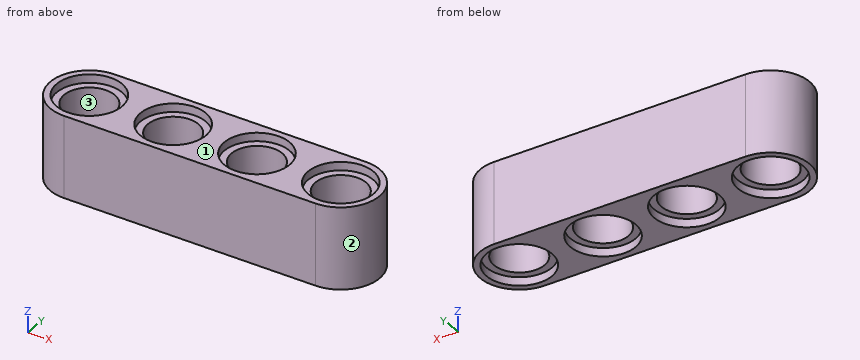
from build123d import *

# Parameters (mm, degrees)
BOSS_EXTRUDE1_DEPTH = 7.76
SKETCH2_R           = 3.1
CUT_EXTRUDE1_DEPTH  = 0.8
SKETCH3_R           = 2.4
CUT_EXTRUDE2_DEPTH  = 93.711483407
CUT_EXTRUDE3_START  = -0.8
SKETCH4_R           = 3.1
CUT_EXTRUDE3_DEPTH  = 0.8


with BuildPart() as part:
    # Sketch1 → Boss-Extrude1 (new body)
    with BuildSketch(Plane.XY):
        with BuildLine():
            Line((-88.686195286, 3.69), (-64.766195286, 3.69))
            ThreePointArc((-64.766195286, 3.69), (-61.076195286, 0), (-64.766195286, -3.69))
            Line((-64.766195286, -3.69), (-88.686195286, -3.69))
            ThreePointArc((-88.686195286, -3.69), (-92.376195286, 0), (-88.686195286, 3.69))
        make_face()
    extrude(amount=BOSS_EXTRUDE1_DEPTH)

    # Sketch2 → Cut-Extrude1 (cut)
    with BuildSketch(Plane(origin=(0, 0, 0), x_dir=(-1, 0, 0), z_dir=(0, 0, -1))):
        with Locations((64.766195286, 0)):
            Circle(SKETCH2_R)
        with Locations((72.736195286, 0)):
            Circle(SKETCH2_R)
        with Locations((80.706195286, 0)):
            Circle(SKETCH2_R)
        with Locations((88.676195286, 0)):
            Circle(SKETCH2_R)
    extrude(amount=-CUT_EXTRUDE1_DEPTH, mode=Mode.SUBTRACT)

    # Sketch3 → Cut-Extrude2 (cut, through all)
    with BuildSketch(Plane(origin=(0, 0, 0.8), x_dir=(-1, 0, 0), z_dir=(0, 0, -1))):
        with Locations((64.766195286, 0)):
            Circle(SKETCH3_R)
        with Locations((72.736195286, 0)):
            Circle(SKETCH3_R)
        with Locations((80.706195286, 0)):
            Circle(SKETCH3_R)
        with Locations((88.676195286, 0)):
            Circle(SKETCH3_R)
    extrude(amount=-CUT_EXTRUDE2_DEPTH, mode=Mode.SUBTRACT)

    # Sketch4 → Cut-Extrude3 (cut)
    with BuildSketch(Plane.XY.offset(7.76).offset(CUT_EXTRUDE3_START)):
        with Locations(Location((-88.676195286, 0, 0), (0, 0, 180))):
            Circle(SKETCH4_R)
        with Locations(Location((-80.706195286, 0, 0), (0, 0, 180))):
            Circle(SKETCH4_R)
        with Locations(Location((-72.736195286, 0, 0), (0, 0, 180))):
            Circle(SKETCH4_R)
        with Locations(Location((-64.766195286, 0, 0), (0, 0, 180))):
            Circle(SKETCH4_R)
    extrude(amount=CUT_EXTRUDE3_DEPTH, mode=Mode.SUBTRACT)


solid = part.part
Part model, mm, in its own coordinate system. Face numbers are marked on the shaded views. Round coordinates to 2 decimals unless told otherwise and drop trailing zeros. Write each loop counter-clockwise with the first axis right and the second up, starting at its lowest first coordinate (ties: lowest second). Pieces come first, ordered by that corner, then holes. Notation, with made-up numbers: M 14,42.5 L 73,42.5 A31 ccw 73,66.5 Z; hole C 25.25,56 d8. An arc over 180 degrees is marked long. Return JSON: item names as keys, results as strings. Group by question number.
(1) Saw through at A-A on z = 3.5. Write the cut outline in (x, y), then the cut area to 3 significant figures.
(2) Drill centre lines: probe 1 along X at (y, z) = (-1, 6.25); probe 2 along Z at (x, y) = (-73, -3); probe 3 along X at (y, z) = (2, 1.5). Where is each one in solid material? Low to high.
(3) Saw through at D-D on x = -70. Write the cut outline in (y, z), then the cut area to 3 significant figures.
(4) Saw through at C-C on y = 0. Count the separate pieces of the cut face and the enclosed holes in it, then the cut area to 3 significant figures.
(5) Saw through at B-B on x = -80. Write the cut outline in (y, z).
(6) Pin check, flat tips, straight feed: pin 1 Ø1.9 at (x, y) = (-88, -0.5) entering from +Z; pin 2 Ø1 at (y, z) = (-2.5, 3.5) entering from +X; pin 3 Ø2 at (y, z) = (2, 4) entering from -X; pin 4 Ø1.9 at (x, y) = (-71.5, 1) entering from -Z. Stop position of each tip, or through.
(7) Two-plate mould, pull along X, no slides. Class the marked faces 1, 2 and 3: +X half, -X half, draft (parallel to the pull), parting line (faces both ways), or undercut.
Returned:
{
 "1": {"outline": "M -88.69,-3.69 L -64.77,-3.69 A3.69 ccw -64.77,3.69 L -88.69,3.69 A3.69 ccw Z; hole C -88.68,0 d4.8; hole C -80.71,0 d4.8; hole C -72.74,0 d4.8; hole C -64.77,0 d4.8", "area": "147 mm²"},
 "2": {"probe 1": "-92.24 to -90.86, -86.49 to -82.89, -78.52 to -74.92, -70.55 to -66.95, -62.58 to -61.21", "probe 2": "0.8 to 6.96", "probe 3": "-91.79 to -90, -87.35 to -82.03, -79.38 to -74.06, -71.41 to -66.09, -63.44 to -61.67"},
 "3": {"outline": "M -3.69,0 L -1.46,0 L -1.46,0.8 L 1.46,0.8 L 1.46,0 L 3.69,0 L 3.69,7.76 L 1.46,7.76 L 1.46,6.96 L -1.46,6.96 L -1.46,7.76 L -3.69,7.76 Z", "area": "52.6 mm²"},
 "4": {"separate pieces": "5", "enclosed holes": "0", "area": "84.9 mm²"},
 "5": {"outline": "M -3.69,0 L -3.02,0 L -3.02,0.8 L -2.29,0.8 L -2.29,6.96 L -3.02,6.96 L -3.02,7.76 L -3.69,7.76 Z; M 2.29,0.8 L 3.02,0.8 L 3.02,0 L 3.69,0 L 3.69,7.76 L 3.02,7.76 L 3.02,6.96 L 2.29,6.96 Z"},
 "6": {"pin 1": "through", "pin 2": "x = -61.67", "pin 3": "x = -92.24", "pin 4": "z = 0.8"},
 "7": {"face 1": "draft", "face 2": "+X half", "face 3": "undercut"}
}
